Geometry: final body of the model. Coordinates: model frame, mm. Give positions to 0.01 mm unless a question says otherwise; leave off trailing zeros. Write each loop counter-clockwise with the first axis right and the second up, starting at its lowest first coordinate (ties: lowest second). Pieces come first, ordered by that corner, then holes.
Autodesk Inventor part; units mm, degrees
ref_plane "YZ Plane" through (0, 0, 0) normal (1, 0, 0) x (0, 1, 0)
ref_plane "XZ Plane" through (0, 0, 0) normal (0, 1, 0) x (-1, 0, 0)
ref_plane "XY Plane" through (0, 0, 0) normal (0, 0, 1) x (1, 0, 0)
sketch "Sketch1" plane through (0, 0, 0) normal (1, 0, 0) x (0, 1, 0)
  point P0 (0, 0)
sketch "Sketch2" plane through (0, 0, 0) normal (1, 0, 0) x (0, 1, 0)
  line L0 (0, 0) -> (0, -22.5)
  line L1 (0, 0) -> (14, 0)
  line L2 (0, -22.5) -> (14, -22.5)
  line L3 (14, 0) -> (14, -1.588)
  line L4 (14, -1.588) -> (1.588, -1.588)
  line L5 (1.588, -1.588) -> (1.588, -20.912)
  line L6 (1.588, -20.912) -> (14, -20.912)
  line L7 (14, -20.912) -> (14, -22.5)
  dimension "d0" = 22.5
  dimension "d1" = 14
  dimension "d2" = 14
  dimension "d3" = 1.588
  dimension "d4" = 12.412
  dimension "d5" = 19.324
extrude "Extrusion1" add sketch "Sketch2" along normal blind 334.01
properties part number "alCchannel"
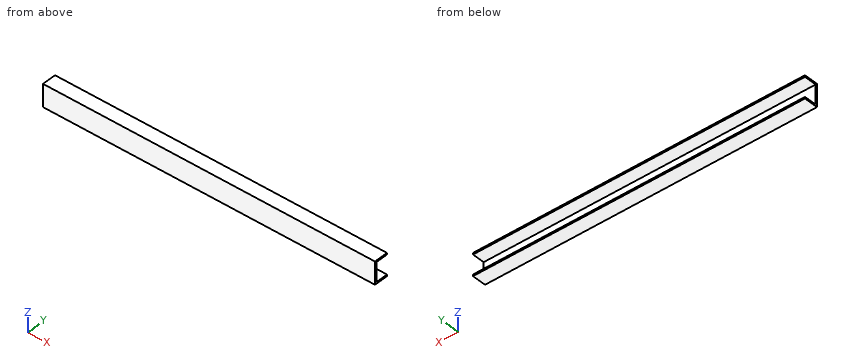
Q1. Section C-C on z = -13.75. Output: boundary loops of the cut face in (x, y), plus the area to 3 significant figures.
Filled sheet:
outline: (0, 0) - (334.01, 0) - (334.01, 1.59) - (0, 1.59) - close
area: 530 mm2
Q2. Ray query, line 1 along Z through (x, y) = (26, 9.5); line 2 along Y through (x, z) = (310, -14.5). Return the intervals inside material, ascending.
Filled sheet:
line 1: z = -22.5 to -20.91, -1.59 to 0
line 2: y = 0 to 1.59
Q3. Section B-B on x = 70. Output: boundary loops of the cut face in (y, z).
Filled sheet:
outline: (0, -22.5) - (14, -22.5) - (14, -20.91) - (1.59, -20.91) - (1.59, -1.59) - (14, -1.59) - (14, 0) - (0, 0) - close
Q4. Section A-A on y = 9.25. Output: boundary loops of the cut face in (x, z), plus the area to 3 significant figures.
Filled sheet:
outline: (0, -22.5) - (334.01, -22.5) - (334.01, -20.91) - (0, -20.91) - close; (0, -1.59) - (334.01, -1.59) - (334.01, 0) - (0, 0) - close
area: 1,060 mm2
Q5. Pin query (flat end, axial travel): P1, Ø5, axis at y = 2, z = -13.5, coming from the +X side; P2, Ø4, axis at x = 253, z = -10, coming from the +Y side. Return the tip coordinate at first contact, or that it passes through.
Filled sheet:
P1: stops at x = 334.01
P2: stops at y = 1.59
